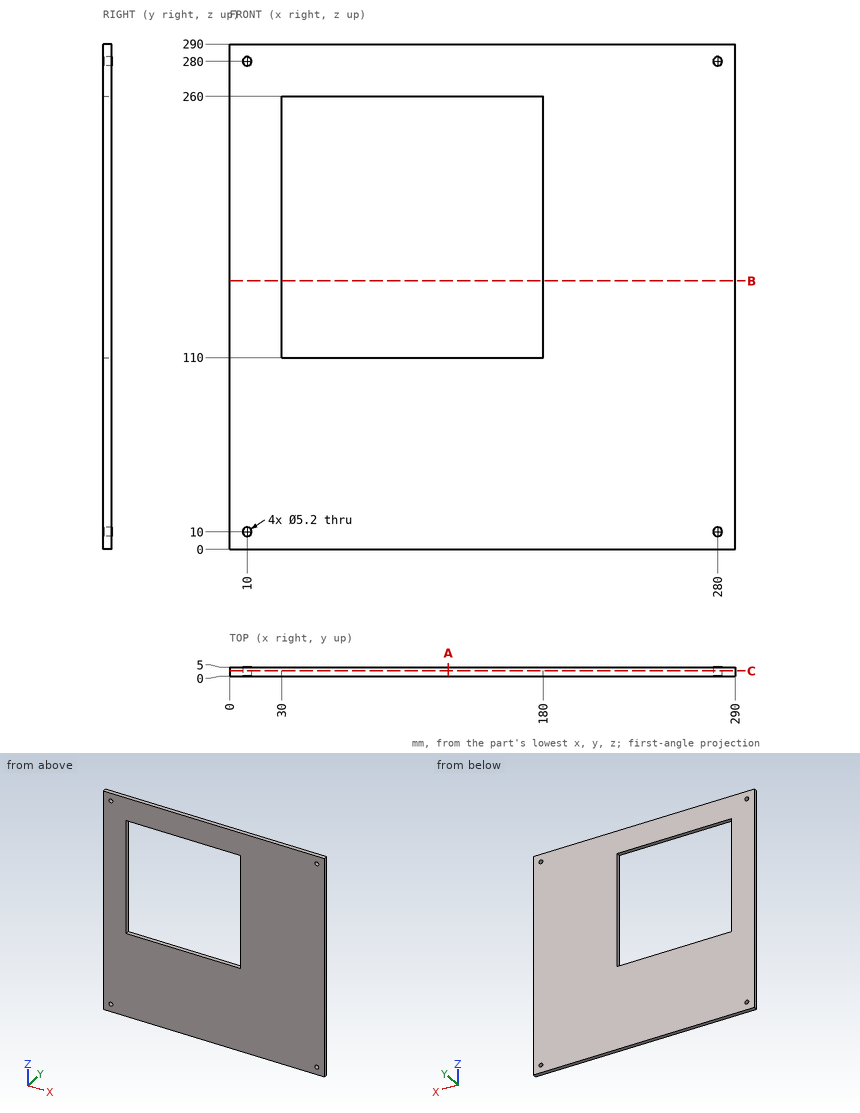
Design review of the part shown in the three views and the two pictorial views. Dimensions are in mm from the part's minimum x, y and z. Coordinates: 2 decimals unless noted, no trailing zeros. Loops run counter-clockwise (first coordinate to the right, second up) from the corner with the lowest first, then second, coordinate; pieces in that order, holes last. Notation, with made-up numbers: M 47,-10 L 101,-10 A35 cw 101,25 Z; hole C 12,37 d9. An arc over 180 degrees is marked long. One line per question, with ' | ' between items.
(1) We need section C-C (y = 3). Give the boundary of the cut face in (x, z), and give its area (3 significant figures).
Filled in:
outline: M 0,0 L 290,0 L 290,290 L 0,290 Z; hole C 10,10 d5.2; hole C 10,280 d5.2; hole M 30,110 L 180,110 L 180,260 L 30,260 Z; hole C 280,10 d5.2; hole C 280,280 d5.2 | area: 61,500 mm^2
(2) Wall thickness on probe 1 along X at (y, z) = (1.2, 10); probe 2 along Z at (x, y) = (157.5, 4.3): over which ranges is each line inside the solid? List them lowest first.
Filled in:
probe 1: x = 0 to 7.4, 12.6 to 277.4, 282.6 to 290 | probe 2: z = 0 to 110, 260 to 290
(3) We need section B-B (z = 154). Give the boundary of the cut face in (x, y).
Filled in:
outline: M 0,0 L 30,0 L 30,5 L 0,5 Z; M 180,0 L 290,0 L 290,5 L 180,5 Z
(4) We need section A-A (x = 125.5). Give the boundary of the cut face in (y, z), and give its area (3 significant figures).
Filled in:
outline: M 0,0 L 5,0 L 5,110 L 0,110 Z; M 0,260 L 5,260 L 5,290 L 0,290 Z | area: 700 mm^2
